Autodesk Inventor part; units mm, degrees
ref_plane "YZ Plane" through (0, 0, 0) normal (1, 0, 0) x (0, 1, 0)
ref_plane "XZ Plane" through (0, 0, 0) normal (0, 1, 0) x (-1, 0, 0)
ref_plane "XY Plane" through (0, 0, 0) normal (0, 0, 1) x (1, 0, 0)
sketch "Sketch1" plane through (0, 0, 0) normal (0, 1, 0) x (-1, 0, 0)
  line L0 (10, 31.05) -> (-10, 31.05)
  line L1 (-10, 31.05) -> (-10, -10)
  line L2 (-10, -10) -> (10, -10)
  line L3 (10, -10) -> (10, 31.05)
  point P0 (0, 0)
  dimension "d0" = 20
  dimension "d1" = 41.05
extrude "Extrusion1" add sketch "Sketch1" along normal blind 2
sketch "Sketch2" plane through (0, 2, 0) normal (0, 1, 0) x (1, 0, 0)
  line L0 (-10, -31.05) -> (10, -31.05)
  line L1 (0, -31.05) -> (-6.35, -31.05)
  line L2 (-6.35, -20.15) -> (6.35, -20.15)
  line L3 (6.35, -31.05) -> (0, -31.05)
  line L4 (10, 10) -> (-10, 10)
  line L5 (-6.35, -0.9) -> (6.35, -0.9)
  line L6 (-6.35, 10) -> (6.35, 10)
  line L7 (-6.35, -31.05) -> (-10, -31.05)
  line L8 (-10, 10) -> (-10, -31.05)
  line L9 (-10, -20.15) -> (-6.35, -20.15)
  line L10 (6.35, -31.05) -> (10, -31.05)
  line L11 (10, -31.05) -> (10, 10)
  line L12 (10, -20.15) -> (6.35, -20.15)
  line L13 (6.35, -0.9) -> (10, -0.9)
  line L14 (10, 10) -> (6.35, 10)
  line L15 (10, -0.9) -> (10, 10)
  line L16 (10, -31.05) -> (10, -20.15)
  line L17 (-10, -31.05) -> (-10, -20.15)
  line L18 (-6.35, -0.9) -> (-10, -0.9)
  line L19 (-10, -0.9) -> (-10, 10)
  line L20 (-10, 10) -> (-6.35, 10)
  point P0 (0, 0)
  dimension "d4" = 6.35
  dimension "d5" = 10.9
  dimension "d6" = 12.7
  dimension "d7" = 10.9
extrude "Extrusion2" add sketch "Sketch2" along normal blind 48.3354 contours L8 L9 L2 L12 L11 L0 | L8 L4 L11 L13 L5 L18
sketch "Sketch9" plane through (-10, 0, 31.05) normal (0, 0, 1) x (1, 0, 0)
  arc A0 (15.084, 42.3223) -> (4.684, 42.3223) centre (9.884, 42.3223) ccw
  line L0 (15.084, 35.9247) -> (15.084, 42.3223)
  line L1 (4.684, 41.1247) -> (4.684, 42.3223)
  arc A1 (15.084, 42.3223) -> (4.684, 42.3223) centre (9.884, 42.3223) ccw
  line L2 (4.684, 42.3223) -> (4.684, 35.9247)
  line L3 (9.8827, 20.3222) -> (-0.0013, 20.3222)
  line L4 (-0.0013, 30.726) -> (-0.0013, 20.3222)
  line L5 (4.684, 35.9247) -> (4.684, 30.726)
  line L6 (15.084, 35.9247) -> (15.0853, 25.5254)
  arc A2 (15.084, 35.9247) -> (15.084, 35.9251) centre (9.884, 35.9243) ccw
  line L7 (4.684, 30.726) -> (-0.0013, 30.726)
  arc A3 (9.8827, 20.3222) -> (15.0853, 25.5254) centre (9.8827, 25.5248) ccw
  point P0 (10, 0)
fillet "Fillet4" radius 10 4 edges at (10, 50.3354, 25.6) (-10, 50.3354, 25.6) (-10, 50.3354, -4.55) (10, 50.3354, -4.55)
sketch "Sketch10" plane through (0, 2, 0) normal (0, 1, 0) x (1, 0, 0)
  line L0 (10, -31.05) -> (-10, -31.05)
  line L1 (-10, 10) -> (10, 10)
  line L2 (10, -20.15) -> (10, -0.9)
  line L3 (-10, -0.9) -> (-10, -20.15)
  line L4 (10, -10.525) -> (-10, -10.525)
  circle A0 centre (0, -10.525) radius 3.302
  point P0 (0, 0)
  dimension "d53" = 41.05
  dimension "d54" = 6.604
extrude "Extrusion10" cut sketch "Sketch10" against normal blind 2
extrude "Extrusion11" cut sketch "Sketch9" against normal through all
properties part number "6 Backet Adjustment"
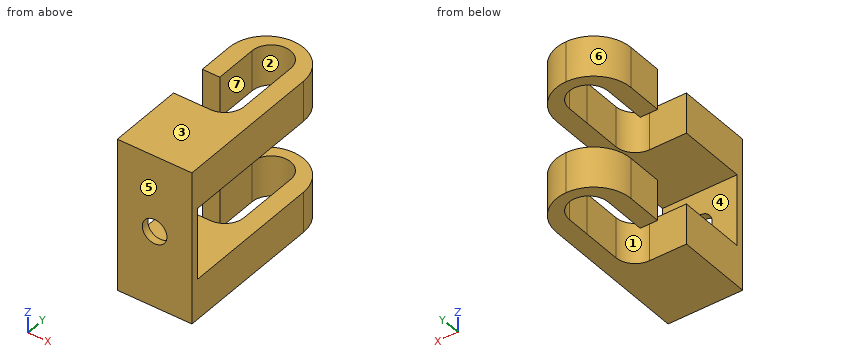
The model under review builds one solid part; all positions refer to its coordinate system, in mm. Face numbers are marked on the shaded views. A direction names the side the tool comes from. Give positions to 0.01 mm unless a question says otherwise; leave off trailing zeros. Order: outer loops, then holes, each group sorted by start corner. A loop starts at its lowest first (then second) coordinate and runs counter-clockwise, first axis right, second up. Notation, with made-up numbers: M 31,72.25 L 56,72.25 A21 ccw 56,80.25 Z; hole C -6,-11 d8. An arc over 180 degrees is marked long. Answer in a Markdown table with one row per item. Add a question column.
1. Mouldability with a two-part tool opening along Y and no side actions: class the marked faces 5, 6 and 7 as released by +Y, released by -Y, zero draft, split by the parting line, or undercut.
2. For pin 1 Ø6 at (x, z) = (-3, 14) entering from +Y; pin 2 Ø2 at (x, z) = (-5.5, 21) entering from +Y; pin 3 Ø5 at (x, z) = (-6, 24.5) entering from +Y, all flat-tipped, find the tip position at first contact; note any pin that passes through.
3. Add section B-B on y = 37. State the section outline as (x, z) points.
4. Add section C-C on z = 12. State the section outline as (x, y) points, plus the area to 3 significant figures.
5. Machinability: for the marked faces 1, 2, 3 and 4, which of the approach directions +Z, -Z, +X, -X, +Y, -Y give a long, thin tool a straight path to every point of the face, cutting with its end or side? Answer none if there is none.
6. Add section A-A on y = 5.5. State the section outline as (x, z) points, plus the area to 3 significant figures.
7. To check wall thickness, follow line 1 along X through (y, z) = (39, 22); line 2 along Z through (x, y) = (0, 1.5); line 3 along Z through (x, y) = (8, 28). State the ranges of each line that lie inside material, in increasing order.
The answers:
| question | item | result |
|---|---|---|
| 1 | face 5 | released by -Y |
| 1 | face 6 | released by +Y |
| 1 | face 7 | undercut |
| 2 | pin 1 | y = 2 |
| 2 | pin 2 | y = 49.27 |
| 2 | pin 3 | y = 49.7 |
| 3 | outline | M -10,-10 L -5.32,-10 L -5.32,0.9 L -10,0.9 Z; M -10,20.15 L -5.32,20.15 L -5.32,31.05 L -10,31.05 Z; M 5.08,-10 L 10,-10 L 10,0.9 L 5.08,0.9 Z; M 5.08,20.15 L 10,20.15 L 10,31.05 L 5.08,31.05 Z |
| 4 | outline | M -10,0 L -2.95,0 L -2.95,2 L -10,2 Z; M 2.95,0 L 10,0 L 10,2 L 2.95,2 Z |
| 4 | area | 28.2 mm2 |
| 5 | face 1 | +Z, -Z, -X |
| 5 | face 2 | +Z, -Z |
| 5 | face 3 | +Z, +X, -X, +Y, -Y |
| 5 | face 4 | +X, -X, +Y |
| 6 | outline | M -10,-10 L 10,-10 L 10,0.9 L -10,0.9 Z; M -10,20.15 L 10,20.15 L 10,31.05 L -10,31.05 Z |
| 6 | area | 436 mm2 |
| 7 | line 1 | -10 to -5.32, 5.08 to 10 |
| 7 | line 2 | -10 to 7.22, 13.83 to 31.05 |
| 7 | line 3 | -10 to 0.9, 20.15 to 31.05 |
